Work out the finished part from the listing and answer in its coordinate system (mm). A direction names the side the tool comes from. Give positions to 0.01 mm unless a question says otherwise; leave off trailing zeros. Loops run counter-clockwise (first coordinate to the right, second up) from the corner with the lowest first, then second, coordinate; pieces in that order, holes last. Notation, with made-up numbers: (-31.75, 70.25) -> (-25.75, 70.25) arc R10 cw to (-25.75, 74.25) -> close; hole circle Ø11 at (14, 72.25). An arc over 180 degrees is marked (long way). Answer as CSV lines item,"result". Start each with the question number.
1. Find the intervals of material crossed by line 1 along Z through (x, y) = (-11, -1.25); line 2 along X through (y, z) = (-10, 9.5); line 3 along X through (y, z) = (-21.75, 8.25), in increasing order.
2. Determine the mould class of faces 1 (the face through (0, 0, 3)), 2 (the face through (-3.264, -12.325, 10.551)), 3 (the face through (11.194, -12.675, 12.013)) for opening direction X: +X half, -X half, draft (parallel to the pull), parting line (faces both ways), or undercut.
3. Find section A-A, the plane z = 8. Give the vertices of the cut face in (x, y), and give its area (3 significant figures).
4. Flat-ended cylindrical pins translate along their axes: pin 1 Ø1.5 at (y, z) = (-16.5, 2) entering from -X; pin 2 Ø3 at (y, z) = (-18.5, 3) entering from -X; pin 3 Ø6.5 at (x, y) = (5, -9.5) entering from +Z. Find the tip coordinate at first contact, or state that the pin passes through.
5. A tool of negligible diameter and unlimited length cuts with its end or side. For faces 4 (the face through (-9, -12, 4)), 5 (the face through (0, -25, 3)), 6 (the face through (4, -12, 4)), from which of +Z, -Z, +X, -X, +Y, -Y can it reach the whole face along a straight path? Write none if from no direction.
6. Find section D-D, the plane z = -1. Give the vertices of the cut face in (x, y).
7. Find section B-B, the plane y = -17. Give the vertices of the cut face in (x, z).
8. Find section C-C, the plane x = 3. Give the vertices of the cut face in (y, z).
from build123d import *

# Parameters (mm, degrees)
F1_DEPTH    = 25
F2_R        = 5
F3_T1_DEPTH = 60.7481164893
F3_T3_DEPTH = 50
F4_R        = 5


# Not quite as in the source:
# - a fillet or chamfer that OpenCascade refuses, or shapes differently, is made with other operations: its cross-section is extruded or revolved along the edge and cut away or added


with BuildPart() as f1:
    # F0 (on Front) → F1 (new body)
    with BuildSketch(Plane.XZ):
        Polygon((-16, -4), (16, -4), (16, 4), (8, 4), (0, 4), (-8, 4), (-16, 4), align=None)
        Polygon((8, 4), (16, 4), (11.6250231628, 12.7824456607), (3.6250231628, 12.7824456607), align=None)
        Polygon((-16, 20.0594142323), (-8, 4), (0, 4), (-8, 20.0594142323), align=None)
    extrude(amount=F1_DEPTH)

    # F2
    f2_edges = [f1.edges().sort_by_distance(p)[0] for p in [
        (-8, -12.5, 20.059414),
        (11.625023, -12.5, 12.782446),
        (16, -12.5, 4),
    ]]
    fillet(f2_edges, radius=F2_R)

    # F3: fillet of radius 5 on 4 edges, made by hand

    # F3_s2 → F3_t1 (cut)
    with BuildSketch(Plane.XZ.offset(-17.8740582446)):
        with BuildLine():
            ThreePointArc((8.529734301, 12.7824456607), (6.4591533037, 9.9078621452), (6.812957963, 6.3828999728))
            Line((6.812957963, 6.3828999728), (3.6250231628, 12.7824456607))
            Line((3.6250231628, 12.7824456607), (8.529734301, 12.7824456607))
        make_face()
        with BuildLine():
            ThreePointArc((-12.8120651998, 13.6598685445), (-13.1658698591, 17.1848307168), (-11.0952888618, 20.0594142323))
            Line((-11.0952888618, 20.0594142323), (-16, 20.0594142323))
            Line((-16, 20.0594142323), (-12.8120651998, 13.6598685445))
        make_face()
    extrude(amount=F3_T1_DEPTH, mode=Mode.SUBTRACT)

    # F3_s4 → F3_t3 (cut)
    with BuildSketch(Plane.XZ.offset(-12.5)):
        with BuildLine():
            ThreePointArc((-16, -1), (-14.5355339059, 2.5355339059), (-11, 4))
            Line((-11, 4), (-16, 4))
            Line((-16, 4), (-16, -1))
        make_face()
        with BuildLine():
            ThreePointArc((-11, -4), (-14.5355339059, -2.5355339059), (-16, 1))
            Line((-16, 1), (-16, -4))
            Line((-16, -4), (-11, -4))
        make_face()
    extrude(amount=F3_T3_DEPTH, mode=Mode.SUBTRACT)

    # F4
    f4_edges = [f1.edges().sort_by_distance(p)[0] for p in [
        (16, -12.5, -4),
    ]]
    fillet(f4_edges, radius=F4_R)


solid = f1.part
Resolved:
1,line 1,"z = -4 to 4, 10.02 to 20.06"
1,line 2,"x = -10.74 to -2.74, 6.37 to 13.26"
1,line 3,"x = -10.12 to -2.12, 6.3 to 13.88"
2,face 1,"draft"
2,face 2,"undercut"
2,face 3,"+X half"
3,outline,"(-9.99, -25) -> (-1.99, -25) -> (-1.99, 0) -> (-9.99, 0) -> close; (6.33, -25) -> (14.01, -25) -> (14.01, 0) -> (6.33, 0) -> close"
3,area,"392 mm^2"
4,pin 1,"stops at x = -15.47"
4,pin 2,"stops at x = -15.33"
4,pin 3,"stops at z = 12.58"
5,face 4,"-X, +Y, -Y"
5,face 5,"+Z, -Z, +X, -X, -Y"
5,face 6,"+Y, -Y"
6,outline,"(-15.58, -25) -> (15.58, -25) -> (15.58, 0) -> (-15.58, 0) -> close"
7,outline,"(-15.9, 0) arc R5 ccw to (-11, -4) -> (11, -4) arc R5 ccw to (16, 1) -> (16, 2.82) arc R5 ccw to (15.48, 5.05) -> (13.01, 10.01) arc R5 ccw to (8.53, 12.78) arc R5 ccw to (6.81, 6.38) -> (8, 4) -> (0, 4) -> (-6.62, 17.29) arc R5 ccw to (-11.1, 20.06) arc R5 ccw to (-12.81, 13.66) -> (-8, 4) -> (-11, 4) arc R5 ccw to start"
8,outline,"(-25, -4) -> (0, -4) -> (0, 4) -> (-25, 4) -> close"
